```python
from build123d import *

# Parameters (mm, degrees)
SKETCH_1_R             = 18.5
EXTRUDE_1_DEPTH        = 24
SKETCH_2_R             = 16.5
EXTRUDE_2_DEPTH        = 22.7
SKETCH_3_R             = 6
EXTRUDE_3_DEPTH        = 6
SKETCH_4_R             = 3
EXTRUDE_4_DEPTH        = 15.5
SKETCH_5_W             = 5.944067487
SKETCH_5_H             = 2.922499848
CUT_EXTRUDE_1_DEPTH    = 12
HOLE_WIZARD_M3_1_D     = 2.5
HOLE_WIZARD_M3_1_DEPTH = 7.5
HOLE_WIZARD_M3_1_TIP   = 0.751075774


with BuildPart() as part:
    # 草图1 → 凸台-拉伸1 (new body)
    with BuildSketch(Plane.XY):
        Circle(SKETCH_1_R)
    extrude(amount=EXTRUDE_1_DEPTH)

    # 草图2 → 凸台-拉伸2 (add)
    with BuildSketch(Plane.XY.offset(24)):
        Circle(SKETCH_2_R)
    extrude(amount=EXTRUDE_2_DEPTH)

    # 草图3 → 凸台-拉伸3 (add)
    with BuildSketch(Plane(origin=(0, 0, 0), x_dir=(-1, 0, 0), z_dir=(0, 0, -1))):
        with Locations((0, 7)):
            Circle(SKETCH_3_R)
    extrude(amount=EXTRUDE_3_DEPTH)

    # 草图4 → 凸台-拉伸4 (add)
    with BuildSketch(Plane(origin=(0, 0, -6), x_dir=(-1, 0, 0), z_dir=(0, 0, -1))):
        with Locations((0, 7)):
            Circle(SKETCH_4_R)
    extrude(amount=EXTRUDE_4_DEPTH)

    # 草图5 → 切除-拉伸1 (cut)
    with BuildSketch(Plane(origin=(0, 0, -21.5), x_dir=(-1, 0, 0), z_dir=(0, 0, -1))):
        with Locations((0.222902531, 10.961249924)):
            Rectangle(SKETCH_5_W, SKETCH_5_H)
    extrude(amount=-CUT_EXTRUDE_1_DEPTH, mode=Mode.SUBTRACT)

    # M3 螺纹孔1
    with Locations(Plane(origin=(0, 0, 0), x_dir=(-1, 0, 0), z_dir=(0, 0, -1))):
        with Locations((-15.5, 0), (-7.75, 13.423393759), (7.75, 13.423393759), (15.5, 0), (7.75, -13.423393759), (-7.75, -13.423393759)):
            Hole(HOLE_WIZARD_M3_1_D / 2, depth=HOLE_WIZARD_M3_1_DEPTH)
            with Locations((0, 0, -(HOLE_WIZARD_M3_1_DEPTH + HOLE_WIZARD_M3_1_TIP / 2))):  # 118° drill point
                Cone(0, HOLE_WIZARD_M3_1_D / 2, HOLE_WIZARD_M3_1_TIP, mode=Mode.SUBTRACT)


solid = part.part
```
The listing builds one solid part. Answer for the finished solid, in the listing's coordinates (mm). A direction names the side the tool comes from. Coordinates: 2 decimals unless noted, no trailing zeros. Loops run counter-clockwise (first coordinate to the right, second up) from the corner with the lowest first, then second, coordinate; pieces in that order, holes last. Notation, with made-up numbers: M 82,-9 L 113,-9 A19 cw 113,20 Z; hole C 39,-30.75 d8. An arc over 180 degrees is marked long. Answer as CSV lines item,"result". Start each with the question number.
(1) The part is cut by section A-A (x = -12). Give the vertices of the cut face in (y, z).
(2) The mould has two halves that part along X. Classify faces 5 (the cylindrical face through (-8.67, 14.27, 3.8)), 6 (the cylindrical face through (0.78, 12.95, -2.96)), 7 (the flat face through (0, 7, -21.5)), 8 (the conical face through (7.91, -13.28, 8.12)): pulls with the +X half, pulls with the -X half, needs draft (parallel to the pull), parting line crosses it, or undercut.
(3) Find the intervals of material crossed by L1, parallel to Y at x = 7, z = 4; L2, parallel to Z at x = -16, y = 7; L3, parallel to Y at x = 0.5, z = 24.5, in increasing order. Write a range as [from, to].
(4) For faces 1 (the cylindrical face through (15.24, -6.32, 35.19)), 2 (the flat face through (0, 0, 46.7)), 3 (the cylindrical face through (0.65, 4.07, -13.64)), 4 (the flat face through (0, 9.5, -16)), determine the directions among +Z, -Z, +X, -X, +Y, -Y from which every point of the face is accessible in a straight line to the end or side of a thin tool.
(5) The part is cut by section B-B (y = 7). Give the vertices of the cut face in (x, z), and give its area (3 significant figures).
(6) Given pin 1 (5 mm diameter, centred on x = -1.5, z = 4.5, fed in from -Y); pin 2 (3 mm diameter, centred on x = 7.75, y = 13.42, fed in from -Z); pin 3 (1.5 mm diameter, centred on x = -1.5, z = -11.5, fed in from -Y), each flat-ended and moving along its own axis, determine where each tip first touches the part or whether it passes through.
(7) The part is cut by section C-C (z = 15.5). Give the vertices of the cut face in (x, y), and give its area (3 significant figures).
(8) The part is cut by section D-D (y = -2.5). Give the vertices of the cut face in (x, z).
Determined:
1,outline,"M -14.08,0 L 14.08,0 L 14.08,24 L 11.32,24 L 11.32,46.7 L -11.32,46.7 L -11.32,24 L -14.08,24 Z"
2,face 5,"undercut"
2,face 6,"parting line crosses it"
2,face 7,"needs draft"
2,face 8,"undercut"
3,L1,"[-17.12, -14.42], [-12.42, 12.42], [14.42, 17.12]"
3,L2,"[0, 24]"
3,L3,"[-16.49, 16.49]"
4,face 1,"+Z"
4,face 2,"+Z, +X, -X, +Y, -Y"
4,face 3,"-Z"
4,face 4,"-Z, +X, -X, +Y"
5,outline,"M -17.12,0 L -6,0 L -6,-6 L -3,-6 L -3,-21.5 L 3,-21.5 L 3,-6 L 6,-6 L 6,0 L 17.12,0 L 17.12,24 L 14.94,24 L 14.94,46.7 L -14.94,46.7 L -14.94,24 L -17.12,24 Z"
5,area,"1,670 mm2"
6,pin 1,"y = -18.5"
6,pin 2,"z = 0"
6,pin 3,"y = 4.1"
7,outline,"C 0,0 d37"
7,area,"1,080 mm2"
8,outline,"M -18.33,0 L 18.33,0 L 18.33,24 L 16.31,24 L 16.31,46.7 L -16.31,46.7 L -16.31,24 L -18.33,24 Z"
